Design review of the part built by this model. Coordinates are the model's own, in mm. Give positions to 0.01 mm unless a question says otherwise; leave off trailing zeros. Order: outer loops, then holes, each group sorted by start corner. A loop starts at its lowest first (then second) coordinate and runs counter-clockwise, first axis right, second up. Notation, with made-up numbers: (63.25, 6.5) -> (117.25, 6.5) arc R20 ccw to (117.25, 45.5) -> close; hole circle Ø11 at (72.5, -35). An arc over 180 degrees is marked (long way). One line per item, written item: value. Start each with the question number.
1) Consider section C-C (z = -1.4). State the section outline as (x, y) points.
2) Consider section A-A (y = 5). State the section outline as (x, z) points, plus the area to 3 significant figures.
3) For pin 1 (1.5 mm diameter, centred on x = 1, y = 6.5, fed in from +Z), flat-tipped, find the tip position at first contact; note if it passes through.
4) Wall thickness on line 1 along X through (y, z) = (4.75, -1.35); line 2 along Z through (x, y) = (1.35, 0.75); line 3 along Y through (x, z) = (-1, -1.15): over which ranges is each line inside the solid? List them lowest first. Write a range as from..to.
5) Consider section D-D (z = -0.35). State the section outline as (x, y) points.
6) Consider section B-B (x = -1.1). State the section outline as (y, z) points, plus the area to 3 significant figures.
from build123d import *

# Parameters (mm, degrees)
SKETCH1_W           = 2.54
SKETCH1_H           = 2.54
MAIN_BODY_DEPTH     = 7.112
CUT_EXTRUDE_3_DEPTH = 7.112
SKETCH2_W           = 0.64
SKETCH2_H           = 0.64
CUT_EXTRUDE_4_DEPTH = 6.35


with BuildPart() as part:
    # Sketch1 → Main Body (new body)
    with BuildSketch(Plane(origin=(0, 0, 0), x_dir=(1, 0, 0), z_dir=(0, 1, 0))):
        with Locations((1.27, 1.27)):
            Rectangle(SKETCH1_W, SKETCH1_H)
    main_body = extrude(amount=MAIN_BODY_DEPTH)

    # Sketch4 → Вырез-Вытянуть3 (cut)
    with BuildSketch(Plane(origin=(0, 0, 0), x_dir=(1, 0, 0), z_dir=(0, 1, 0))):
        Polygon((2.54, 2.54), (2.286, 2.54), (2.54, 2.032), align=None)
        Polygon((2.54, 0), (2.286, 0), (2.54, 0.508), align=None)
    cut_extrude_3 = extrude(amount=CUT_EXTRUDE_3_DEPTH, mode=Mode.SUBTRACT)

    # Sketch2 → Вырез-Вытянуть4 (cut)
    with BuildSketch(Plane(origin=(0, 0, 0), x_dir=(1, 0, 0), z_dir=(0, 1, 0))):
        with Locations((1.27, 1.27)):
            Rectangle(SKETCH2_W, SKETCH2_H)
    cut_extrude_4 = extrude(amount=CUT_EXTRUDE_4_DEPTH, mode=Mode.SUBTRACT)

    # Зеркальное отражение1: Main Body, Вырез-Вытянуть3, Вырез-Вытянуть4 across Right Plane
    add(main_body.mirror(Plane(origin=(0, 0, 0), x_dir=(0, 0, -1), z_dir=(1, 0, 0))))
    add(cut_extrude_3.mirror(Plane(origin=(0, 0, 0), x_dir=(0, 0, -1), z_dir=(1, 0, 0))), mode=Mode.SUBTRACT)
    add(cut_extrude_4.mirror(Plane(origin=(0, 0, 0), x_dir=(0, 0, -1), z_dir=(1, 0, 0))), mode=Mode.SUBTRACT)


solid = part.part
Checked values:
1. outline: (-2.54, 0) -> (-1.59, 0) -> (-1.59, 6.35) -> (-0.95, 6.35) -> (-0.95, 0) -> (0.95, 0) -> (0.95, 6.35) -> (1.59, 6.35) -> (1.59, 0) -> (2.54, 0) -> (2.54, 7.11) -> (-2.54, 7.11) -> close
2. outline: (-2.54, -2.03) -> (-2.29, -2.54) -> (2.29, -2.54) -> (2.54, -2.03) -> (2.54, -0.51) -> (2.29, 0) -> (-2.29, 0) -> (-2.54, -0.51) -> close; hole (-1.59, -1.59) -> (-0.95, -1.59) -> (-0.95, -0.95) -> (-1.59, -0.95) -> close; hole (0.95, -1.59) -> (1.59, -1.59) -> (1.59, -0.95) -> (0.95, -0.95) -> close
2. area: 11.8 mm^2
3. pin 1: stops at z = 0
4. line 1: x = -2.54..-1.59, -0.95..0.95, 1.59..2.54
4. line 2: z = -2.54..-1.59, -0.95..0
4. line 3: y = 6.35..7.11
5. outline: (-2.46, 0) -> (2.46, 0) -> (2.46, 7.11) -> (-2.46, 7.11) -> close
6. outline: (0, -2.54) -> (7.11, -2.54) -> (7.11, 0) -> (0, 0) -> (0, -0.95) -> (6.35, -0.95) -> (6.35, -1.59) -> (0, -1.59) -> close
6. area: 14.0 mm^2
